```python
from build123d import *

# Parameters (mm, degrees)
SKETCH1_W                    = 38.1
SKETCH1_H                    = 38.1
BOSS_EXTRUDE1_DEPTH          = 79.375
SKETCH3_R                    = 8.5725
CUT_EXTRUDE1_DEPTH           = 10.35812
CUT_EXTRUDE1_DRAFT           = -1.783333333
LPATTERN1_COUNT              = 4
LPATTERN1_PITCH              = 38.1
LPATTERN1_COPY_1_SKETCH_R    = 8.5725
LPATTERN1_COPY_1_DEPTH       = 10.35812
LPATTERN1_COPY_1_DRAFT       = -1.783333333
LPATTERN1_COPY_2_SKETCH_R    = 8.5725
LPATTERN1_COPY_2_DEPTH       = 10.35812
LPATTERN1_COPY_2_DRAFT       = -1.783333333
LPATTERN1_COPY_3_SKETCH_R    = 8.5725
LPATTERN1_COPY_3_DEPTH       = 10.35812
LPATTERN1_COPY_3_DRAFT       = -1.783333333
SKETCH8_R                    = 10.668
CUT_EXTRUDE3_DEPTH           = 11.721742741
CUT_EXTRUDE3_DRAFT           = -1.783333333
SKETCH13_R                   = 11.064875
CUT_EXTRUDE6_DEPTH           = 2.54
CUT_EXTRUDE6_TAPER           = 45
CUT_EXTRUDE6_OTHER_WAY_DEPTH = 10.16
CUT_EXTRUDE6_OTHER_WAY_TAPER = 45
CIRPATTERN2_COUNT            = 2
CIRPATTERN2_COPY_1_SKETCH_R  = 10.668
CIRPATTERN2_COPY_1_DEPTH     = 11.721742741
CIRPATTERN2_COPY_1_DRAFT     = -1.783333333
SKETCH12_R                   = 2.54
CUT_EXTRUDE5_DEPTH           = 91.082757178
CIRPATTERN3_COUNT            = 2
CIRPATTERN3_ANGLE            = 90


# Read off the part's stored shape, not the designer's step: Cut-Extrude2
with BuildPart() as part:
    # Sketch1 → Boss-Extrude1 (new, symmetric)
    with BuildSketch(Plane.XY):
        Rectangle(SKETCH1_W, SKETCH1_H)
    extrude(amount=BOSS_EXTRUDE1_DEPTH, both=True)

    # Sketch2 → Cut-Revolve1 (revolve, cut)
    with BuildSketch(Plane(origin=(0, 0, 0), x_dir=(0, 0, -1), z_dir=(1, 0, 0)), mode=Mode.PRIVATE) as cut_revolve1_sk:
        Polygon((57.15, 19.05), (57.15, -4.411631326), (64.4921875, 0), (64.4921875, 19.05), align=None)
    cut_revolve1 = revolve(cut_revolve1_sk.sketch.rotate(Axis((0, 26.3921875, -57.15), (0, -1, 0)), 180), axis=Axis((0, 26.3921875, -57.15), (0, -1, 0)), mode=Mode.SUBTRACT)


with BuildPart() as cut_extrude1_tool:
    # Sketch3 → Cut-Extrude1 (with draft: the straight prism first)
    with BuildSketch(Plane(origin=(0, 19.05, 0), x_dir=(1, 0, 0), z_dir=(0, 1, 0))):
        with Locations((0, 57.15)):
            Circle(SKETCH3_R)
    extrude(amount=-CUT_EXTRUDE1_DEPTH)
    # Cut-Extrude1: the draft: its side faces are tilted about the plane it starts from
    cut_extrude1_sides = [cut_extrude1_tool.faces().sort_by_distance(p)[0] for p in [
        (-8.5725, 13.87094, -57.15),
    ]]
    draft(cut_extrude1_sides, Plane(origin=(0, 19.05, 0), x_dir=(1, 0, 0), z_dir=(0, 1, 0)), CUT_EXTRUDE1_DRAFT)


with BuildPart() as part_1:
    add(part.part)

    # Cut-Extrude1: cut by cut_extrude1_tool
    add(cut_extrude1_tool.part, mode=Mode.SUBTRACT)

    # Cut-Extrude2 outline → Cut-Extrude2 (revolve, cut)
    with BuildSketch(Plane.XY.offset(-57.15)):
        Polygon((8.567591048, 19.05), (8.567591048, 18.892333789), (8.725257259, 19.05), align=None)
    cut_extrude2 = revolve(axis=Axis((0, 0, -57.15), (0, 1, 0)), mode=Mode.SUBTRACT)

    # LPattern1: Cut-Revolve1, Cut-Extrude2 ×4
    with Locations(*[(0, 0, i * LPATTERN1_PITCH) for i in range(1, LPATTERN1_COUNT)]):
        add(cut_revolve1, mode=Mode.SUBTRACT)
        add(cut_extrude2, mode=Mode.SUBTRACT)


with BuildPart() as lpattern1_copy_1_tool:
    # LPattern1 copy 1 sketch → LPattern1 copy 1 (with draft: the straight prism first)
    with BuildSketch(Plane(origin=(0, 19.05, 38.1), x_dir=(1, 0, 0), z_dir=(0, 1, 0))):
        with Locations((0, 57.15)):
            Circle(LPATTERN1_COPY_1_SKETCH_R)
    extrude(amount=-LPATTERN1_COPY_1_DEPTH)
    # LPattern1 copy 1: the draft: its side faces are tilted about the plane it starts from
    lpattern1_copy_1_sides = [lpattern1_copy_1_tool.faces().sort_by_distance(p)[0] for p in [
        (-8.5725, 13.87094, -19.05),
    ]]
    draft(lpattern1_copy_1_sides, Plane(origin=(0, 19.05, 38.1), x_dir=(1, 0, 0), z_dir=(0, 1, 0)), LPATTERN1_COPY_1_DRAFT)


with BuildPart() as part_2:
    add(part_1.part)

    # LPattern1 copy 1: cut by lpattern1_copy_1_tool
    add(lpattern1_copy_1_tool.part, mode=Mode.SUBTRACT)


with BuildPart() as lpattern1_copy_2_tool:
    # LPattern1 copy 2 sketch → LPattern1 copy 2 (with draft: the straight prism first)
    with BuildSketch(Plane(origin=(0, 19.05, 76.2), x_dir=(1, 0, 0), z_dir=(0, 1, 0))):
        with Locations((0, 57.15)):
            Circle(LPATTERN1_COPY_2_SKETCH_R)
    extrude(amount=-LPATTERN1_COPY_2_DEPTH)
    # LPattern1 copy 2: the draft: its side faces are tilted about the plane it starts from
    lpattern1_copy_2_sides = [lpattern1_copy_2_tool.faces().sort_by_distance(p)[0] for p in [
        (-8.5725, 13.87094, 19.05),
    ]]
    draft(lpattern1_copy_2_sides, Plane(origin=(0, 19.05, 76.2), x_dir=(1, 0, 0), z_dir=(0, 1, 0)), LPATTERN1_COPY_2_DRAFT)


with BuildPart() as part_3:
    add(part_2.part)

    # LPattern1 copy 2: cut by lpattern1_copy_2_tool
    add(lpattern1_copy_2_tool.part, mode=Mode.SUBTRACT)


with BuildPart() as lpattern1_copy_3_tool:
    # LPattern1 copy 3 sketch → LPattern1 copy 3 (with draft: the straight prism first)
    with BuildSketch(Plane(origin=(0, 19.05, 114.3), x_dir=(1, 0, 0), z_dir=(0, 1, 0))):
        with Locations((0, 57.15)):
            Circle(LPATTERN1_COPY_3_SKETCH_R)
    extrude(amount=-LPATTERN1_COPY_3_DEPTH)
    # LPattern1 copy 3: the draft: its side faces are tilted about the plane it starts from
    lpattern1_copy_3_sides = [lpattern1_copy_3_tool.faces().sort_by_distance(p)[0] for p in [
        (-8.5725, 13.87094, 57.15),
    ]]
    draft(lpattern1_copy_3_sides, Plane(origin=(0, 19.05, 114.3), x_dir=(1, 0, 0), z_dir=(0, 1, 0)), LPATTERN1_COPY_3_DRAFT)


with BuildPart() as part_4:
    add(part_3.part)

    # LPattern1 copy 3: cut by lpattern1_copy_3_tool
    add(lpattern1_copy_3_tool.part, mode=Mode.SUBTRACT)

    # Sketch7 → Cut-Revolve2 (revolve, cut)
    with BuildSketch(Plane(origin=(0, 0, 0), x_dir=(0, 0, -1), z_dir=(1, 0, 0)), mode=Mode.PRIVATE) as cut_revolve2_sk:
        Polygon((-79.375, 0), (5.484730838, 0), (0, 9.128125), (-79.375, 9.128125), align=None)
    cut_revolve2 = revolve(cut_revolve2_sk.sketch.rotate(Axis((0, 0, 88.503125), (0, 0, -1)), 90), axis=Axis((0, 0, 88.503125), (0, 0, -1)), mode=Mode.SUBTRACT)


with BuildPart() as cut_extrude3_tool:
    # Sketch8 → Cut-Extrude3 (with draft: the straight prism first)
    with BuildSketch(Plane.XY.offset(79.375)):
        Circle(SKETCH8_R)
    extrude(amount=-CUT_EXTRUDE3_DEPTH)
    # Cut-Extrude3: the draft: its side faces are tilted about the plane it starts from
    cut_extrude3_sides = [cut_extrude3_tool.faces().sort_by_distance(p)[0] for p in [
        (-10.668, 0, 73.514128629),
    ]]
    draft(cut_extrude3_sides, Plane.XY.offset(79.375), CUT_EXTRUDE3_DRAFT)


with BuildPart() as part_5:
    add(part_4.part)

    # Cut-Extrude3: cut by cut_extrude3_tool
    add(cut_extrude3_tool.part, mode=Mode.SUBTRACT)

    # Sketch13 → Cut-Extrude6 (cut)
    with BuildSketch(Plane.XY.offset(79.375)):
        Circle(SKETCH13_R)
    cut_extrude6 = extrude(amount=-CUT_EXTRUDE6_DEPTH, taper=CUT_EXTRUDE6_TAPER, mode=Mode.SUBTRACT)

    # Sketch13 → Cut-Extrude6 other way (cut)
    with BuildSketch(Plane.XY.offset(79.375)):
        Circle(SKETCH13_R)
    extrude(amount=CUT_EXTRUDE6_OTHER_WAY_DEPTH, taper=CUT_EXTRUDE6_OTHER_WAY_TAPER, mode=Mode.SUBTRACT)

    # CirPattern2: Cut-Revolve2, Cut-Extrude6 ×2 about axis
    cirpattern2_axis = Axis((0, 21.367211937, 0), (0, -1, 0))
    add([cut_revolve2.rotate(cirpattern2_axis, i * 360 / CIRPATTERN2_COUNT) for i in range(1, CIRPATTERN2_COUNT)], mode=Mode.SUBTRACT)
    add([cut_extrude6.rotate(cirpattern2_axis, i * 360 / CIRPATTERN2_COUNT) for i in range(1, CIRPATTERN2_COUNT)], mode=Mode.SUBTRACT)


with BuildPart() as cirpattern2_copy_1_tool:
    # CirPattern2 copy 1 sketch → CirPattern2 copy 1 (with draft: the straight prism first)
    with BuildSketch(Plane(origin=(0, 0, -79.375), x_dir=(-1, 0, 0), z_dir=(0, 0, -1))):
        Circle(CIRPATTERN2_COPY_1_SKETCH_R)
    extrude(amount=-CIRPATTERN2_COPY_1_DEPTH)
    # CirPattern2 copy 1: the draft: its side faces are tilted about the plane it starts from
    cirpattern2_copy_1_sides = [cirpattern2_copy_1_tool.faces().sort_by_distance(p)[0] for p in [
        (10.668, 0, -73.514128629),
    ]]
    draft(cirpattern2_copy_1_sides, Plane(origin=(0, 0, -79.375), x_dir=(-1, 0, 0), z_dir=(0, 0, -1)), CIRPATTERN2_COPY_1_DRAFT)


with BuildPart() as part_6:
    add(part_5.part)

    # CirPattern2 copy 1: cut by cirpattern2_copy_1_tool
    add(cirpattern2_copy_1_tool.part, mode=Mode.SUBTRACT)

    # Sketch12 → Cut-Extrude5 (cut, through all)
    with BuildSketch(Plane(origin=(0, 19.05, 0), x_dir=(1, 0, 0), z_dir=(0, 1, 0))):
        with Locations(Location((-14.224, 38.1, 0), (0, 0, 270))):
            Circle(SKETCH12_R)
        with Locations(Location((14.224, -38.1, 0), (0, 0, 270))):
            Circle(SKETCH12_R)
    cut_extrude5 = extrude(amount=-CUT_EXTRUDE5_DEPTH, mode=Mode.SUBTRACT)

    # CirPattern3: Cut-Extrude5 ×2 about axis
    cirpattern3_axis = Axis((0, 0, 87.593551009), (0, 0, 1))
    for i in range(1, CIRPATTERN3_COUNT):
        add(cut_extrude5.rotate(cirpattern3_axis, i * CIRPATTERN3_ANGLE / (CIRPATTERN3_COUNT - 1)), mode=Mode.SUBTRACT)


solid = part_6.part
```
Source: CAD feature listing. Evaluate the final solid. Frame: model axes, mm. A direction names the side the tool comes from. Coordinates: 2 decimals unless noted, no trailing zeros. Loops run counter-clockwise (first coordinate to the right, second up) from the corner with the lowest first, then second, coordinate; pieces in that order, holes last. Notation, with made-up numbers: M 61.5,4.25 L 99.5,4.25 A21 cw 99.5,41.25 Z; hole C -8.75,-17.5 d9. An arc over 180 degrees is marked long. Use a Markdown table: item, result. Add a question column.
Q1. Draft query along Z for faces 1 (the flat face through (0, -19.05, 1)), 2 (the flat face through (8, 9, -79.375)), 3 (the cylindrical face through (-7.34, 7.44, 19.17)). Return one class per face: pulls with the +Z half, pulls with the -Z half, needs draft (parallel to the pull), parting line crosses it, or undercut.
Q2. Section query B-B, the plane z = 19.05. Return loops of the section in (x, y), and give its area (3 significant figures).
Q3. First-contact query: pin 1 (2.5 mm diameter, centred on x = -6, z = 59, fed in from +Y); pin 2 (2.5 mm diameter, centred on x = 5.5, z = -18, fed in from +Y); pin 3 (4.5 mm diameter, centred on x = -5, z = 19.5, fed in from +Y). Flat tips, straight axial feed; report the tip coordinate or a pass-through.
Q4. Material intervals for L1, parallel to Z at x = 14, y = -9 (3 decimals); L2, parallel to X at y = 6, z = 38.1; L3, parallel to X at y = 6, z = -72, sorted ascending.
Q5. Access query for faces 4 (the cylindrical face through (-7.34, 7.44, 57.27)), 5 (the conical face through (-9.998, 3.148, -73.388)), 6 (the cylindrical face through (11.744, -2.18, 37.549)). Directions: +Z, -Z, +X, -X, +Y, -Y. A direction counts if a zero-diameter tool reaches every point of the face in a straight line with its end or side. Return the directions, or none.
Q6. Section query C-C, the plane x = -0.5. State how many separate pieces and enclosed holes the cut face has, and give its area (3 significant figures).
Q7. Section query A-A, the plane z = -38.1. Return loops of the section in (x, y), and give its area (3 significant figures).
Result:
| question | item | result |
|---|---|---|
| 1 | face 1 | needs draft |
| 1 | face 2 | pulls with the -Z half |
| 1 | face 3 | undercut |
| 2 | outline | M -19.05,-19.05 L 19.05,-19.05 L 19.05,19.05 L 8.73,19.05 L 8.57,18.89 L 8.25,8.69 L 7.34,8.69 L 7.34,5.42 A9.13 cw long -7.34,5.42 L -7.34,8.69 L -8.25,8.69 L -8.57,18.89 L -8.73,19.05 L -19.05,19.05 Z |
| 2 | area | 1,010 mm2 |
| 3 | pin 1 | stops at y = 8.69 |
| 3 | pin 2 | stops at y = -6.14 |
| 3 | pin 3 | stops at y = -5.55 |
| 4 | L1 | z = -79.375 to 35.57, 40.63 to 79.375 |
| 4 | L2 | x = -19.05 to -6.88, 6.88 to 11.68, 16.76 to 19.05 |
| 4 | L3 | x = -19.05 to -8.54, 8.54 to 19.05 |
| 5 | face 4 | +Y |
| 5 | face 5 | -Z |
| 5 | face 6 | +Y, -Y |
| 6 | separate pieces | 6 |
| 6 | enclosed holes | 2 |
| 6 | area | 2,380 mm2 |
| 7 | outline | M -19.05,-19.05 L -16.76,-19.05 L -16.76,-16.76 L -19.05,-16.76 Z; M -19.05,-11.68 L -16.76,-11.68 L -16.76,19.05 L -19.05,19.05 Z; M -11.68,-19.05 L 19.05,-19.05 L 19.05,-16.76 L -11.68,-16.76 Z; M -11.68,-11.68 L 19.05,-11.68 L 19.05,19.05 L -11.68,19.05 Z; hole C 0,0 d18.26 |
| 7 | area | 829 mm2 |
